The listing builds one solid part. Answer for the finished solid, in the listing's coordinates (mm). Coordinates: 2 decimals unless noted, no trailing zeros. Write each loop counter-clockwise with the first axis right and the second up, starting at its lowest first coordinate (ties: lowest second). Pieces come first, ordered by that corner, then holes.
from build123d import *

# Parameters (mm, degrees)
SKETCH1_R           = 13.5
BOSS_EXTRUDE1_DEPTH = 5
SKETCH2_R           = 5
BOSS_EXTRUDE2_DEPTH = 2
SKETCH3_R           = 1.5
CUT_EXTRUDE1_DEPTH  = 8
CHAMFER1_SIZE       = 2


with BuildPart() as part:
    # Sketch1 → Boss-Extrude1 (new body)
    with BuildSketch(Plane.XY):
        Circle(SKETCH1_R)
    extrude(amount=BOSS_EXTRUDE1_DEPTH)

    # Sketch2 → Boss-Extrude2 (add)
    with BuildSketch(Plane.XY.offset(5)):
        Circle(SKETCH2_R)
    extrude(amount=BOSS_EXTRUDE2_DEPTH)

    # Sketch3 → Cut-Extrude1 (cut, through all)
    with BuildSketch(Plane.XY.offset(7)):
        Circle(SKETCH3_R)
    extrude(amount=-CUT_EXTRUDE1_DEPTH, mode=Mode.SUBTRACT)

    # Chamfer1
    chamfer1_edges = [part.edges().sort_by_distance(p)[0] for p in [
        (-1.5, 0, 0),
    ]]
    chamfer(chamfer1_edges, length=CHAMFER1_SIZE)


solid = part.part
Q1. The part is cut by section C-C, the plane z = 1.5. Write down the section's boundary in (x, y).
Answers below:
outline: circle Ø27 at (0, 0); hole circle Ø4 at (0, 0)
Q2. Find the intervals of material crossed by probe 1 along Y at (x, z) = (0, 5.9); probe 2 along Y at (x, z) = (0, 3.6); probe 3 along Z at (x, y) = (11.25, 7), in increasing order.
Answers below:
probe 1: y = -5 to -1.5, 1.5 to 5
probe 2: y = -13.5 to -1.5, 1.5 to 13.5
probe 3: z = 0 to 5
Q3. The part is cut by section A-A, the plane x = 0. Write down the section's boundary in (y, z), then the cut area to 3 significant figures.
Answers below:
outline: (-13.5, 0) - (-3.5, 0) - (-1.5, 2) - (-1.5, 7) - (-5, 7) - (-5, 5) - (-13.5, 5) - close; (1.5, 2) - (3.5, 0) - (13.5, 0) - (13.5, 5) - (5, 5) - (5, 7) - (1.5, 7) - close
area: 130 mm2
Q4. Determine the mould class of faces 1 (the face through (-1.5, 0.07, 4.54)), 2 (the face through (-1.08, -4.88, 5.99)), 3 (the face through (6, 0, 5)) for opening direction Y: released by +Y, released by -Y, zero draft, split by the parting line, or undercut.
Answers below:
face 1: undercut
face 2: split by the parting line
face 3: zero draft
Q5. Given pin 1 (1.5 mm diameter, centred on x = -4, z = 2, fed in from +Y); pin 2 (1 mm diameter, centred on y = 3.5, z = 1.5, fed in from -X); pin 3 (4 mm diameter, centred on x = 5.5, z = 5, fed in from -Y), each flat-ended and moving along its own axis, determine where each tip first touches the part or whether it passes through.
Answers below:
pin 1: stops at y = 13.1
pin 2: stops at x = -13.16
pin 3: stops at y = -13.04
Q6. The part is cut by section D-D, the plane y = 8. Write down the section's boundary in (x, z), then the cut area to 3 significant figures.
Answers below:
outline: (-10.87, 0) - (10.87, 0) - (10.87, 5) - (-10.87, 5) - close
area: 109 mm2
